Design review of the part built by this model. Coordinates are the model's own, in mm. Face numbers are marked on the shaded views. A direction names the side the tool comes from. Give positions to 0.01 mm unless a question says otherwise; leave off trailing zeros. Loops run counter-clockwise (first coordinate to the right, second up) from the corner with the lowest first, then second, coordinate; pieces in that order, holes last. Notation, with made-up numbers: (-17.75, 62) -> (-6.75, 62) arc R26 ccw to (-6.75, 98) -> close; hole circle Ø6 at (83, 80.5). An arc over 180 degrees is marked (long way). Answer in a Markdown table with one row per item. Add a question column.
(1) Consider section B-B on z = 6.25. Write out the cut boundary in (x, y), then the cut area to 3 significant figures.
(2) Consider section A-A on y = 5.5. Write out the cut boundary in (x, z).
(3) For the marked faces 1 and 2, list the 3-axis set-ups (+Z, -Z, +X, -X, +Y, -Y) from which the entire face can be reached by the end or side of a thin tool; tool diameter is ignored.
(4) Draft analysis for pull direction X (two halves, no side actions). For the marked faces 3, 4 and 5, state which applies: +X half, -X half, draft (parallel to the pull), parting line (faces both ways), or undercut.
(5) For line 1 (Z direction, x = 24.5, y = 21); line 2 (X direction, y = 19, z = 5.25); line 3 (Z direction, x = 2, y = 18.5), list the stretches that pass through material, from the lowest coordinate up.
(6) For pin 1 (0.8 mm diameter, centred on x = -1, y = 0.5, fed in from -Z); pin 2 (0.8 mm diameter, centred on x = -0.5, y = 1.5, fed in from +Z); pin 3 (0.7 mm diameter, centred on x = -1.27, y = 1.02, fed in from +Z); pin 4 (3.5 mm diameter, centred on y = 14.5, z = 6, fed in from -X), all flat-tipped, find the tip position at first contact; note any pin that passes through.
from build123d import *

# Parameters (mm, degrees)
BOSS_EXTRUDE1_DEPTH = 12.7
FILLET7_R           = 3.048
FILLET8_R           = 1.27
SHELL2_T            = -0.4572
SKETCH2_W           = 7.9502
SKETCH2_H           = 1.016
CUT_EXTRUDE1_DEPTH  = 11.7856
SKETCH4_W           = 1.3462
SKETCH4_H           = 1.5875
SKETCH5_R           = 0.5715
CUT_EXTRUDE2_DEPTH  = 11.3124001


with BuildPart() as part:
    # Sketch1 → Boss-Extrude1 (new body)
    with BuildSketch(Plane.XY):
        with BuildLine():
            Line((0, 0), (38.1, 0))
            Line((38.1, 0), (38.1, 23.2918))
            ThreePointArc((38.1, 23.2918), (19.05, 24.758348548), (0, 23.2918))
            Line((0, 23.2918), (0, 0))
        make_face()
    extrude(amount=BOSS_EXTRUDE1_DEPTH)

    # Fillet7
    fillet7_edges = [part.edges().sort_by_distance(p)[0] for p in [
        (38.1, 11.6459, 12.7),
        (0, 11.6459, 12.7),
        (38.1, 11.6459, 0),
        (0, 11.6459, 0),
    ]]
    fillet(fillet7_edges, radius=FILLET7_R)

    # Fillet8
    fillet8_edges = [part.edges().sort_by_distance(p)[0] for p in [
        (38.1, 23.2918, 6.35),
        (19.05, 24.758348548, 0),
        (0, 23.2918, 6.35),
        (19.05, 24.758348548, 12.7),
        (0.897565394, 23.427470684, 11.812077539),
        (0.897565394, 23.427470684, 0.887922461),
        (37.20243455, 23.427470691, 11.812077599),
        (37.20243455, 23.427470691, 0.887922401),
    ]]
    fillet(fillet8_edges, radius=FILLET8_R)

    # Shell2
    shell2_openings = [part.faces().sort_by_distance(p)[0] for p in [
        (19.05, 0, 6.35),
    ]]
    offset(amount=SHELL2_T, openings=shell2_openings, kind=Kind.INTERSECTION)

    # Sketch2 → Cut-Extrude1 (cut)
    with BuildSketch(Plane.ZY):
        with Locations((6.35, 0.508)):
            Rectangle(SKETCH2_W, SKETCH2_H)
    extrude(amount=-CUT_EXTRUDE1_DEPTH, mode=Mode.SUBTRACT)

    # Sketch4 → Revolve1 (revolve)
    with BuildSketch(Plane.XZ.offset(-1.016)):
        with Locations((-0.597849635, 6.35635)):
            Rectangle(SKETCH4_W, SKETCH4_H)
        with Locations((-0.597849635, 9.53135)):
            Rectangle(SKETCH4_W, SKETCH4_H)
        with Locations((-0.597849635, 3.18135)):
            Rectangle(SKETCH4_W, SKETCH4_H)
    revolve(axis=Axis((-1.270949635, 1.016, 10.3251), (0, 0, -1)))

    # Sketch5 → Cut-Extrude2 (cut, through all)
    with BuildSketch(Plane(origin=(0, 0, 2.3876), x_dir=(-1, 0, 0), z_dir=(0, 0, -1))):
        with Locations((1.270949635, 1.016)):
            Circle(SKETCH5_R)
    extrude(amount=-CUT_EXTRUDE2_DEPTH, mode=Mode.SUBTRACT)


solid = part.part
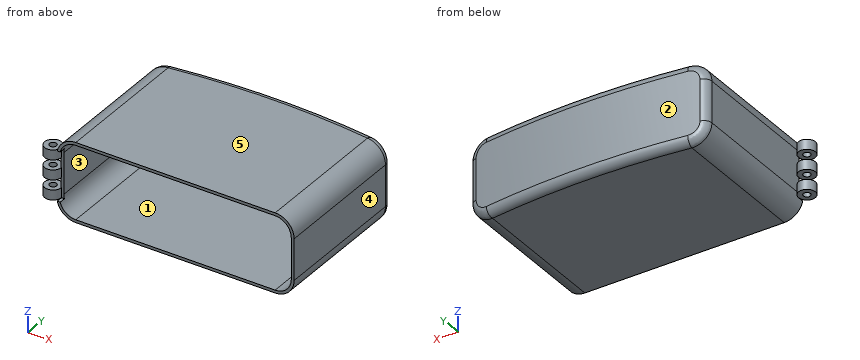
Values follow:
| question | item | result |
|---|---|---|
| 1 | outline | (0, 1.46) arc R1.35 ccw (long way) to (0.08, 1.02) -> (0.46, 1.02) -> (0.46, 22.2) arc R0.81 cw to (1.15, 23) arc R124 cw to (36.95, 23) arc R0.81 cw to (37.64, 22.2) -> (37.64, 0) -> (38.1, 0) -> (38.1, 22.2) arc R1.27 ccw to (37.01, 23.46) arc R124.46 ccw to (1.09, 23.46) arc R1.27 ccw to (0, 22.2) -> close; hole circle Ø1.14 at (-1.27, 1.02) |
| 1 | area | 42.3 mm2 |
| 2 | outline | (0, 3.05) arc R3.05 ccw to (3.05, 0) -> (35.05, 0) arc R3.05 ccw to (38.1, 3.05) -> (38.1, 9.65) arc R3.05 ccw to (35.05, 12.7) -> (3.05, 12.7) arc R3.05 ccw to (0, 9.65) -> close; hole (0.46, 3.05) arc R2.59 ccw to (3.05, 0.46) -> (35.05, 0.46) arc R2.59 ccw to (37.64, 3.05) -> (37.64, 9.65) arc R2.59 ccw to (35.05, 12.24) -> (3.05, 12.24) arc R2.59 ccw to (0.46, 9.65) -> close |
| 3 | face 1 | -Y |
| 3 | face 2 | +Z, -Z, +Y |
| 4 | face 3 | undercut |
| 4 | face 4 | +X half |
| 4 | face 5 | draft |
| 5 | line 1 | 0 to 0.46, 12.24 to 12.7 |
| 5 | line 2 | 0 to 0.46, 37.64 to 38.1 |
| 5 | line 3 | 0.19 to 0.68, 12.02 to 12.51 |
| 6 | pin 1 | z = 2.39 |
| 6 | pin 2 | z = 10.33 |
| 6 | pin 3 | through |
| 6 | pin 4 | x = 0 |
